Geometry: final body of the model. Coordinates: model frame, mm. Give positions to 0.01 mm unless a question says otherwise; leave off trailing zeros. Loops run counter-clockwise (first coordinate to the right, second up) from the corner with the lowest first, then second, coordinate; pieces in that order, holes last.
from build123d import *

# Parameters (mm, degrees)
F1_DEPTH = 184.404
F0_W     = 5.334
F0_H     = 6.35
F2_DEPTH = 6.35
F3_R     = 5.08


with BuildPart() as f1:
    # F0 (on Top) → F1 (new body)
    with BuildSketch(Plane.XY):
        Polygon((9.017, -42.8625), (-9.017, -42.8625), (-2.667, -61.831036), (2.667, -61.831036), align=None)
    extrude(amount=F1_DEPTH)

    # F0 (on Top) → F2 (join)
    with BuildSketch(Plane.XY):
        with Locations((0, -65.006036)):
            Rectangle(F0_W, F0_H)
    extrude(amount=F2_DEPTH)

    # F3
    f3_edges = [f1.edges().sort_by_distance(p)[0] for p in [
        (0, -61.831036, 184.404),
    ]]
    fillet(f3_edges, radius=F3_R)


solid = f1.part
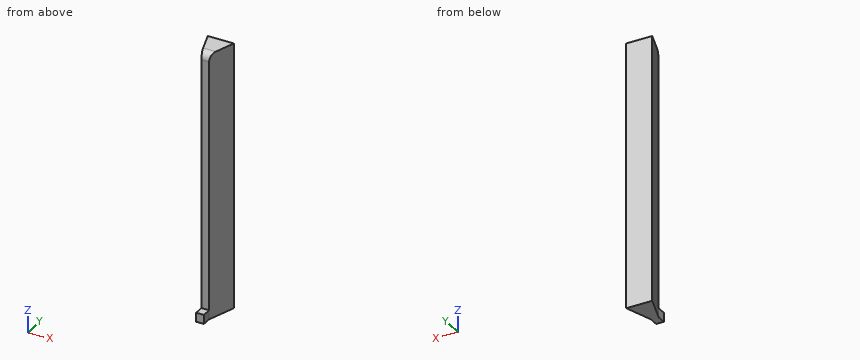
Item 1: Ray query, probe 1 along Z at (x, y) = (2, -62.25); probe 2 along Y at (x, z) = (-0.5, 132); probe 3 along X at (y, z) = (-57.25, 103). Return the intervals inside material, ascending.
Values follow:
probe 1: z = 0 to 6.35
probe 2: y = -61.83 to -42.86
probe 3: x = -4.2 to 4.2
Item 2: Section query B-B on y = -65. Return loops of the section in (x, z).
Values follow:
outline: (-2.67, 0) - (2.67, 0) - (2.67, 6.35) - (-2.67, 6.35) - close
Item 3: Section query A-A on z = 125.5. Return loops of the section in (x, y).
Values follow:
outline: (-9.02, -42.86) - (-2.67, -61.83) - (2.67, -61.83) - (9.02, -42.86) - close
Item 4: Pin query (flat end, axial travel): pin 1 (5 mm diameter, centred on y = -48, z = 70.5, fed in from -X); pin 2 (6 mm diameter, centred on x = -0.5, z = 69.5, fed in from -Y); pin 3 (4 mm diameter, centred on x = 1.5, y = -51, fed in from -Z); pin 4 (12 mm diameter, centred on y = -65, z = 40.5, fed in from -X). Return the tip coordinate at first contact, or that it passes through.
Values follow:
pin 1: stops at x = -8.13
pin 2: stops at y = -61.83
pin 3: stops at z = 0
pin 4: stops at x = -3.61
